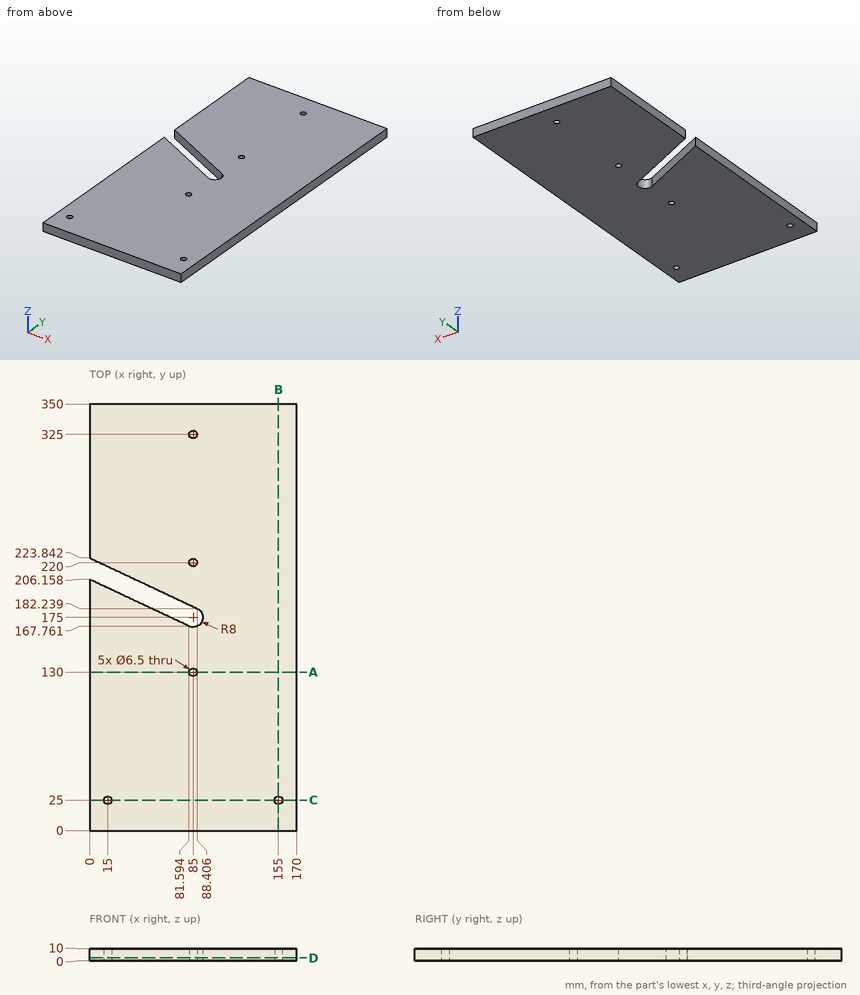
Source: three-view drawing plus pictorial views. Frame: mm from the lowest corner of the part. Give positions to 0.01 mm unless a question says otherwise; leave off trailing zeros. Write each loop counter-clockwise with the first axis right and the second up, starting at its lowest first coordinate (ties: lowest second). Pieces come first, ordered by that corner, then holes. Notation, with made-up numbers: (-3, 22.25) - (47, 22.25) arc R22 ccw to (47, 50.25) - close; hole circle Ø9 at (13, 62). An arc over 180 degrees is marked (long way). Write item = value, one per line. Start each with the question number.
1. Ray query, L1, parallel to X at y = 325, z = 4; L2, parallel to Y at x = 72, z = 2 (1 decimal); L3, parallel to Y at x = 155, z = 6.5. Return the intervals inside material, ascending.
2. Section query A-A, the plane y = 130. Output: boundary loops of the cut face in (x, z), then the cut area to 4 significant figures.
3. Section query B-B, the plane x = 155. Output: boundary loops of the cut face in (y, z).
4. Section query D-D, the plane z = 2.5. Output: boundary loops of the cut face in (x, y), then the cut area to 3 significant figures.
5. Section query C-C, the plane y = 25. Output: boundary loops of the cut face in (x, z), then the cut area to 3 significant figures.
Check sheet entries:
q1.L1 = 0 to 81.75, 88.25 to 170
q1.L2 = 0 to 172.3, 190 to 350
q1.L3 = 0 to 21.75, 28.25 to 350
q2.outline = (0, 0) - (81.75, 0) - (81.75, 10) - (0, 10) - close; (88.25, 0) - (170, 0) - (170, 10) - (88.25, 10) - close
q2.area = 1,635 mm2
q3.outline = (0, 0) - (21.75, 0) - (21.75, 10) - (0, 10) - close; (28.25, 0) - (350, 0) - (350, 10) - (28.25, 10) - close
q4.outline = (0, 0) - (170, 0) - (170, 350) - (0, 350) - (0, 223.84) - (88.41, 182.24) arc R8 cw to (81.59, 167.76) - (0, 206.16) - close; hole circle Ø6.5 at (15, 25); hole circle Ø6.5 at (85, 130); hole circle Ø6.5 at (85, 220); hole circle Ø6.5 at (85, 325); hole circle Ø6.5 at (155, 25)
q4.area = 57,700 mm2
q5.outline = (0, 0) - (11.75, 0) - (11.75, 10) - (0, 10) - close; (18.25, 0) - (151.75, 0) - (151.75, 10) - (18.25, 10) - close; (158.25, 0) - (170, 0) - (170, 10) - (158.25, 10) - close
q5.area = 1,570 mm2
